Input: part model. Units: mm. Frame: model coordinates. A direction names the side the tool comes from. Coordinates: 2 decimals unless noted, no trailing zeros. Loops run counter-clockwise (first coordinate to the right, second up) from the corner with the lowest first, then second, coordinate; pieces in that order, holes last.
Item 1: Pull-direction query (X, two-part tool) for faces 4 (the cylindrical face through (0.49, -7.21, -42.84)), 5 (the flat face through (5, 19.05, -20)), 6 (the flat face through (4.762, 1, -22)); classes: released by +X, released by -X, zero draft, split by the parting line, or undercut.
Item 2: Ray query, line 1 along Z through (x, y) = (-2.75, -13) (3 decimals); line 2 along X through (y, z) = (-14, -16.5); line 3 along Y through (x, z) = (-5.25, -21.5) (3 decimals). Return the intervals inside material, ascending.
Item 3: Reachability of faces 1 (the cylindrical face through (-0.379, 14.595, -42.84)), 2 (the cylindrical face through (-6.127, 17.14, -42.885)), 3 (the flat face through (-2, 2, -41.275)) from +Z, -Z, +X, -X, +Y, -Y: full face, straight path, thin tool, end or side. Return the list, or none.
Item 4: Contact query for flat-ended pins moving along their axis: P1, Ø2, axis at x = -1.5, z = -31.5, coming from the +Y side (3 decimals); P2, Ø5, axis at x = -1.59, y = 12.7, coming from the +Z side; P3, Ø6, axis at y = -7.5, z = -36, coming from the -X side. Output: stop coordinate, or through.
Item 5: Section D-D on x = 1.75. Return loops of the section in (y, z) (3 decimals), and give its area (3 significant figures).
Item 6: Section B-B on x = -0.75. Return loops of the section in (y, z) (3 decimals), and give its area (3 significant figures).
```python
from build123d import *

# Parameters (mm, degrees)
SKETCH1_W           = 15.875
SKETCH1_H           = 38.1
BOSS_EXTRUDE1_DEPTH = 44.45
SHELL1_T            = -3.175
CUT_EXTRUDE1_REACH  = 48.147
SKETCH2_R           = 2.2479
FILLET2_R           = 6.35


with BuildPart() as part:
    # Sketch1 → Boss-Extrude1 (new body)
    with BuildSketch(Plane.XY):
        Rectangle(SKETCH1_W, SKETCH1_H)
    extrude(amount=-BOSS_EXTRUDE1_DEPTH)

    # Shell1
    shell1_openings = [part.faces().sort_by_distance(p)[0] for p in [
        (-7.9375, 0, -22.225),
        (0, 19.05, -22.225),
    ]]
    offset(amount=SHELL1_T, openings=shell1_openings, kind=Kind.INTERSECTION)

    # Sketch2 → Cut-Extrude1 (cut, up to next)
    with BuildSketch(Plane.XY.offset(-3.175), mode=Mode.PRIVATE) as cut_extrude1_sk1:
        with Locations((-1.5875, -6.35)):
            Circle(SKETCH2_R)
    cut_extrude1_tool1 = extrude(cut_extrude1_sk1.sketch, amount=-CUT_EXTRUDE1_REACH, mode=Mode.PRIVATE) & part.part
    # Sketch2 → Cut-Extrude1 (cut, up to next)
    with BuildSketch(Plane.XY.offset(-3.175), mode=Mode.PRIVATE) as cut_extrude1_sk2:
        with Locations((-1.5875, 12.7)):
            Circle(SKETCH2_R)
    cut_extrude1_tool2 = extrude(cut_extrude1_sk2.sketch, amount=-CUT_EXTRUDE1_REACH, mode=Mode.PRIVATE) & part.part
    add(cut_extrude1_tool1.solids().sort_by_distance((-1.5875, -6.35, -3.175))[0], mode=Mode.SUBTRACT)
    add(cut_extrude1_tool2.solids().sort_by_distance((-1.5875, 12.7, -3.175))[0], mode=Mode.SUBTRACT)

    # Fillet2
    fillet2_edges = [part.edges().sort_by_distance(p)[0] for p in [
        (-7.9375, 19.05, -42.8625),
    ]]
    fillet(fillet2_edges, radius=FILLET2_R)


solid = part.part
```
Results found:
1. face 4: undercut
1. face 5: zero draft
1. face 6: released by -X
2. line 1: z = -44.45 to -41.275, -3.175 to 0
2. line 2: x = 4.76 to 7.94
2. line 3: y = -19.05 to -15.875
3. face 1: -Z
3. face 2: -Z, -X, +Y
3. face 3: -X, +Y
4. P1: stops at y = -15.875
4. P2: stops at z = 0
4. P3: stops at x = 4.76
5. outline: (-19.05, -44.45) - (19.05, -44.45) - (19.05, -41.275) - (-15.875, -41.275) - (-15.875, -3.175) - (19.05, -3.175) - (19.05, 0) - (-19.05, 0) - close
5. area: 363 mm2
6. outline: (-19.05, -44.45) - (-8.436, -44.45) - (-8.436, -41.275) - (-15.875, -41.275) - (-15.875, -3.175) - (19.05, -3.175) - (19.05, 0) - (-19.05, 0) - close; (-4.264, -44.45) - (10.614, -44.45) - (10.614, -41.275) - (-4.264, -41.275) - close; (14.786, -44.45) - (19.05, -44.45) - (19.05, -41.275) - (14.786, -41.275) - close
6. area: 336 mm2
